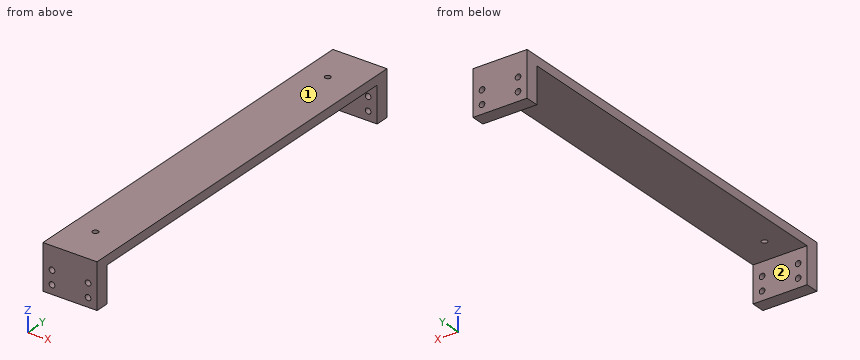
Autodesk Inventor part; units mm, degrees
ref_plane "YZ Plane" through (0, 0, 0) normal (1, 0, 0) x (0, 1, 0)
ref_plane "XZ Plane" through (0, 0, 0) normal (0, 1, 0) x (-1, 0, 0)
ref_plane "XY Plane" through (0, 0, 0) normal (0, 0, 1) x (1, 0, 0)
sketch "스케치1" plane through (0, 0, 0) normal (0, 0, 1) x (1, 0, 0)
  line L0 (-12, 88) -> (12, 88)
  line L1 (12, 88) -> (12, -88)
  line L2 (12, -88) -> (-12, -88)
  line L3 (-12, -88) -> (-12, 88)
  line L4 (-12, 88) -> (12, -88) construction
  line L5 (12, 88) -> (-12, -88) construction
  point P0 (0, 0)
  dimension "d0" = 24
  dimension "d1" = 176
extrude "돌출1" add sketch "스케치1" along normal blind 4
sketch "스케치2" plane through (12, -88, 0) normal (1, 0, 0) x (0, 0, -1)
  line L0 (0, 0) -> (0, 176)
  line L1 (0, 176) -> (-4, 176)
  line L2 (-4, 0) -> (-4, 176)
  line L3 (0, 0) -> (-4, 0)
  line L4 (-4, 0) -> (-4, 176)
  line L5 (-4, 176) -> (16, 176)
  line L6 (16, 176) -> (16, 170)
  line L7 (16, 170) -> (-4, 170)
  line L8 (-4, 170) -> (-4, 176)
  line L9 (-4, 0) -> (16, 0)
  line L10 (16, 0) -> (16, 6)
  line L11 (16, 6) -> (-4, 6)
  line L12 (-4, 6) -> (-4, 0)
  point P0 (0, 88)
  point P1 (0, 6)
  point P2 (0, 170)
  dimension "d4" = 20
  dimension "d5" = 6
  dimension "d6" = 20
  dimension "d7" = 6
extrude "돌출2" add sketch "스케치2" against normal up to surface (24 mm away) contours L0 L11 L10 L9 | L0 L5 L6 L7
sketch "스케치3" plane through (-12, -88, 4) normal (0, -1, 0) x (1, 0, 0)
  line L0 (24, -20) -> (24, 0)
  line L1 (0, 0) -> (24, 0)
  line L2 (0, 0) -> (0, -20)
  line L3 (24, -20) -> (0, -20)
  line L4 (4, -16) -> (4, -4)
  line L5 (4, -4) -> (20, -4)
  line L6 (20, -4) -> (20, -16)
  line L7 (20, -16) -> (4, -16)
  circle A0 centre (20, -16) radius 1.25
  circle A1 centre (4, -16) radius 1.25
  circle A2 centre (20, -4) radius 1.25
  circle A3 centre (4, -4) radius 1.25
  circle A4 centre (20, -10) radius 1.25
  circle A5 centre (4, -10) radius 1.25
  point P0 (12, -4)
  dimension "d10" = 4
  dimension "d11" = 2.5
  dimension "d12" = 2.5
  dimension "d13" = 2.5
  dimension "d14" = 2.5
  dimension "d15" = 2.5
  dimension "d16" = 2.5
extrude "돌출3" cut sketch "스케치3" against normal through all contours L7 A1 L4 | L4 A1 L7 | A5 L4 | L4 A5 | A0 L6 L7 | L7 L6 A0 | A4 L6 | L6 A4
sketch "스케치6" plane through (0, 0, 4) normal (0, 0, 1) x (1, 0, 0)
  circle A0 centre (-1.5, -70.5) radius 1.25
  line L0 (6, -62) -> (6, -79)
  line L1 (-9.5, -79) -> (6, -79)
  line L2 (-9.5, -79) -> (-9.5, -62)
  line L3 (6, -62) -> (-9.5, -62)
  circle A1 centre (-1.5, 70.5) radius 1.25
  line L4 (6, 62) -> (6, 79)
  line L5 (6, 62) -> (-9.5, 62)
  line L6 (-9.5, 79) -> (-9.5, 62)
  line L7 (-9.5, 79) -> (6, 79)
  point P0 (0, 0)
extrude "돌출6" cut sketch "스케치6" against normal blind 10 contours A0 | A1
properties part number "Back_Cover" material "LCP 플라스틱"
Source: CAD feature listing. Evaluate the final solid. Frame: model axes, mm. Face numbers are marked on the shaded views. A direction names the side the tool comes from. Give positions to 0.01 mm unless a question says otherwise; leave off trailing zeros. Write each loop counter-clockwise with the first axis right and the second up, starting at its lowest first coordinate (ties: lowest second). Pieces come first, ordered by that corner, then holes. Notation, with made-up numbers: (83.5, -20) -> (101.5, -20) arc R24 cw to (101.5, -2) -> close; hole circle Ø10 at (1.25, 61.5). An arc over 180 degrees is marked (long way). Return JSON: item names as keys, results as strings. Group by question number.
1. Access query for the marked faces 1 and 2. Directions: +Z, -Z, +X, -X, +Y, -Y. A direction counts if a zero-diameter tool reaches every point of the face in a straight line with its end or side. Return the directions, or none.
2. Material intervals for line 1 (X direction, y = -86.3, z = -6); line 2 (Y direction, x = -5, z = -4.25); line 3 (Z direction, x = -8, y = -85.75), sorted ascending. Write a range as from..to.
3. Section A-A, the plane z = -3.25. Output: boundary loops of the cut face in (x, y).
4. Section B-B, the plane x = -4.75. Output: boundary loops of the cut face in (y, z), then the cut area to 3 significant figures.
5. Pin query (flat end, axial travel): pin 1 Ø1.5 at (x, z) = (-8, -6) entering from -Y; pin 2 Ø3 at (x, y) = (-1.5, 70.5) entering from -Z. Return the tip coordinate at first contact, or that it passes through.
6. Section C-C, the plane y = 50.5. Output: boundary loops of the cut face in (x, z).
Determined:
{
 "1": {"face 1": "+Z, +X, -X, +Y, -Y", "face 2": "-Z, +X, -X"},
 "2": {"line 1": "x = -12..-9.25, -6.75..6.75, 9.25..12", "line 2": "y = -88..-82, 82..88", "line 3": "z = -16..-13.25, -10.75..-7.25, -4.75..4"},
 "3": {"outline": "(-12, -88) -> (12, -88) -> (12, -82) -> (-12, -82) -> close; (-12, 82) -> (12, 82) -> (12, 88) -> (-12, 88) -> close"},
 "4": {"outline": "(-88, -16) -> (-82, -16) -> (-82, 0) -> (82, 0) -> (82, -16) -> (88, -16) -> (88, 4) -> (-88, 4) -> close", "area": "896 mm2"},
 "5": {"pin 1": "passes through", "pin 2": "stops at z = 0"},
 "6": {"outline": "(-12, 0) -> (12, 0) -> (12, 4) -> (-12, 4) -> close"}
}
